CAD build for the part. Positions are in the model's coordinates, mm. A direction names the side the tool comes from. Round coordinates to 2 decimals unless told otherwise and drop trailing zeros. Write each loop counter-clockwise with the first axis right and the second up, starting at its lowest first coordinate (ties: lowest second). Pieces come first, ordered by that corner, then holes. Notation, with made-up numbers: (86, -9.75) -> (135, -9.75) arc R29 ccw to (135, 25.25) -> close; hole circle Ø1 at (77.25, -25.75). An arc over 180 degrees is marked (long way). Answer in a Markdown table with one row per item. Add a question column.
```python
from build123d import *

# Parameters (mm, degrees)
SKETCH028_R   = 2
PAD018_DEPTH  = 3
SKETCH005_R   = 7
PAD003_DEPTH  = 4
FILLET_R      = 1
SKETCH029_R   = 4
SKETCH029_R_2 = 2
PAD019_DEPTH  = 14
SKETCH030_R   = 2
PAD020_DEPTH  = 3
SKETCH031_W   = 18
SKETCH031_H   = 4
PAD021_DEPTH  = 14
SKETCH032_W   = 4
SKETCH032_H   = 18
PAD022_DEPTH  = 14


with BuildPart() as part:
    # Sketch028 (on Face1 of CopySolid004) → Pad018 (new body)
    with BuildSketch(Plane.XY.offset(-16)):
        with BuildLine():
            Line((-7.5, -12.5), (7.5, -12.5))
            ThreePointArc((7.5, -12.5), (11.035534, -11.035534), (12.5, -7.5))
            Line((12.5, -7.5), (12.5, 7.5))
            ThreePointArc((12.5, 7.5), (11.035534, 11.035534), (7.5, 12.5))
            Line((7.5, 12.5), (-7.5, 12.5))
            ThreePointArc((-7.5, 12.5), (-11.035534, 11.035534), (-12.5, 7.5))
            Line((-12.5, 7.5), (-12.5, -7.5))
            ThreePointArc((-12.5, -7.5), (-11.035534, -11.035534), (-7.5, -12.5))
        make_face()
        with Locations((-8, 8)):
            Circle(SKETCH028_R, mode=Mode.SUBTRACT)
        with Locations((8, 8)):
            Circle(SKETCH028_R, mode=Mode.SUBTRACT)
        with Locations((8, -8)):
            Circle(SKETCH028_R, mode=Mode.SUBTRACT)
        with Locations((-8, -8)):
            Circle(SKETCH028_R, mode=Mode.SUBTRACT)
    extrude(amount=PAD018_DEPTH)

    # Sketch005 (on Face13 of Pad018) → Pad003 (join)
    with BuildSketch(Plane(origin=(0, 0, -16), x_dir=(1, 0, 0), z_dir=(0, 0, -1))):
        Circle(SKETCH005_R)
    extrude(amount=PAD003_DEPTH)

    # Fillet
    fillet_edges = [part.edges().sort_by_distance(p)[0] for p in [
        (-7, 0, -20),
    ]]
    fillet(fillet_edges, radius=FILLET_R)

    # Sketch029 (on Face17 of Fillet) → Pad019 (join)
    with BuildSketch(Plane.XY.offset(-13)):
        Circle(SKETCH029_R)
        with Locations((0, 9)):
            Circle(SKETCH029_R_2)
        with Locations((9, 0)):
            Circle(SKETCH029_R_2)
        with Locations((0, -9)):
            Circle(SKETCH029_R_2)
        with Locations((-9, 0)):
            Circle(SKETCH029_R_2)
    extrude(amount=PAD019_DEPTH)

    # Sketch030 (on Face25 of Pad019) → Pad020 (join)
    with BuildSketch(Plane.XY.offset(1)):
        with BuildLine():
            Line((-7.5, -12.5), (7.5, -12.5))
            ThreePointArc((7.5, -12.5), (11.035534, -11.035534), (12.5, -7.5))
            Line((12.5, -7.5), (12.5, 7.5))
            ThreePointArc((12.5, 7.5), (11.035534, 11.035534), (7.5, 12.5))
            Line((7.5, 12.5), (-7.5, 12.5))
            ThreePointArc((-7.5, 12.5), (-11.035534, 11.035534), (-12.5, 7.5))
            Line((-12.5, 7.5), (-12.5, -7.5))
            ThreePointArc((-12.5, -7.5), (-11.035534, -11.035534), (-7.5, -12.5))
        make_face()
        with Locations((-5.656851, 5.656857)):
            Circle(SKETCH030_R, mode=Mode.SUBTRACT)
        with Locations((5.656855, 5.656853)):
            Circle(SKETCH030_R, mode=Mode.SUBTRACT)
        with Locations((5.656855, -5.656853)):
            Circle(SKETCH030_R, mode=Mode.SUBTRACT)
        with Locations((-5.656851, -5.656857)):
            Circle(SKETCH030_R, mode=Mode.SUBTRACT)
    extrude(amount=PAD020_DEPTH)

    # Sketch031 (on Face17 of Pad020) → Pad021 (join)
    with BuildSketch(Plane.XY.offset(-13)):
        Rectangle(SKETCH031_W, SKETCH031_H)
    extrude(amount=PAD021_DEPTH)

    # Sketch032 (on Face17 of Pad021) → Pad022 (join)
    with BuildSketch(Plane.XY.offset(-13)):
        Rectangle(SKETCH032_W, SKETCH032_H)
    extrude(amount=PAD022_DEPTH)


with BuildPart() as part_1:
    # Body010 placement: moved
    add(part.part.moved(Location((0, -99, 8.5))))


solid = part_1.part
```
Item 1: Saw through at C-C on x = 0. Give the cut face in (y, z), then the cut area to 3 significant figures.
Item 2: Drill centre lines: probe 1 along Y at (x, z) = (8, -6.25); probe 2 along Z at (x, y) = (0.5, -110.25); probe 3 along Y at (x, z) = (9.5, -5.25). Where is each one in solid material? Low to high.
Item 3: Pin check, flat tips, straight feed: pin 1 (8 mm diameter, centred on y = -103.5, z = 3, fed in from -X); pin 2 (1.7 mm diameter, centred on x = -7.5, z = 1, fed in from -Y); pin 3 (1.7 mm diameter, centred on y = -92.5, z = 5, fed in from +X). Stop position of each tip, or through.
Item 4: Saw through at B-B on z = 7. Give the cut face in (x, y).
Item 5: Saw through at D-D on y = -99. Give the cut face in (x, z).
Item 6: Two-plate mould, pull along Y, no slides. Class faces 1 (the cylindrical face through (0, -110, 2)), 2 (the cylindrical face through (-5.917, -102.674, 10.979)), 3 (the flat face through (2, -93, 2)): +Y half, -Y half, draft (parallel to the pull), parting line (faces both ways), or undercut.
Item 7: Tool access for faces 4 (the cylindrical face through (-0.91, -105.94, -8.98)), 5 (the flat face through (2, -105, 2)), 6 (the cylindrical face through (-2.839, -101.818, 2.402)): list every direction of +Z, -Z, +X, -X, +Y, -Y with a clear straight run to the whole face (end or side of a thin tool).
Item 8: Saw through at A-A on x = -8. Give the cut face in (y, z).
Recorded:
| question | item | result |
|---|---|---|
| 1 | outline | (-111.5, -7.5) -> (-106, -7.5) -> (-106, -10.5) arc R1 ccw to (-105, -11.5) -> (-93, -11.5) arc R1 ccw to (-92, -10.5) -> (-92, -7.5) -> (-86.5, -7.5) -> (-86.5, -4.5) -> (-88, -4.5) -> (-88, 9.5) -> (-86.5, 9.5) -> (-86.5, 12.5) -> (-111.5, 12.5) -> (-111.5, 9.5) -> (-110, 9.5) -> (-110, -4.5) -> (-111.5, -4.5) -> close |
| 1 | area | 514 mm2 |
| 2 | probe 1 | -111.47 to -109, -105 to -93, -89 to -86.53 |
| 2 | probe 2 | -7.5 to -4.5, 9.5 to 12.5 |
| 2 | probe 3 | -111.08 to -108.32, -105.68 to -92.32, -89.68 to -86.92 |
| 3 | pin 1 | x = -10.94 |
| 3 | pin 2 | y = -101 |
| 3 | pin 3 | x = 2 |
| 4 | outline | (-9, -101) -> (-3.46, -101) arc R4 ccw to (-2, -102.46) -> (-2, -108) arc R2 ccw to (2, -108) -> (2, -102.46) arc R4 ccw to (3.46, -101) -> (9, -101) arc R2 ccw to (9, -97) -> (3.46, -97) arc R4 ccw to (2, -95.54) -> (2, -90) arc R2 ccw to (-2, -90) -> (-2, -95.54) arc R4 ccw to (-3.46, -97) -> (-9, -97) arc R2 ccw to start |
| 5 | outline | (-12.5, -7.5) -> (-7, -7.5) -> (-7, -10.5) arc R1 ccw to (-6, -11.5) -> (6, -11.5) arc R1 ccw to (7, -10.5) -> (7, -7.5) -> (12.5, -7.5) -> (12.5, -4.5) -> (11, -4.5) -> (11, 9.5) -> (12.5, 9.5) -> (12.5, 12.5) -> (-12.5, 12.5) -> (-12.5, 9.5) -> (-11, 9.5) -> (-11, -4.5) -> (-12.5, -4.5) -> close |
| 6 | face 1 | -Y half |
| 6 | face 2 | undercut |
| 6 | face 3 | draft |
| 7 | face 4 | -Z |
| 7 | face 5 | +X, -Y |
| 7 | face 6 | -X, -Y |
| 8 | outline | (-111.47, -7.5) -> (-109, -7.5) -> (-109, -4.5) -> (-111.47, -4.5) -> close; (-111.47, 9.5) -> (-101, 9.5) -> (-101, -4.5) -> (-105, -4.5) -> (-105, -7.5) -> (-93, -7.5) -> (-93, -4.5) -> (-97, -4.5) -> (-97, 9.5) -> (-86.53, 9.5) -> (-86.53, 12.5) -> (-111.47, 12.5) -> close; (-89, -7.5) -> (-86.53, -7.5) -> (-86.53, -4.5) -> (-89, -4.5) -> close |
